```python
from build123d import *

# Parameters (mm, degrees)
SKETCH1_W           = 107.199818646
SKETCH1_H           = 66.816994634
BOSS_EXTRUDE1_DEPTH = 15
SKETCH2_R           = 8.587881919
BOSS_EXTRUDE2_DEPTH = 15
SKETCH3_R           = 13.34182577
BOSS_EXTRUDE3_DEPTH = 80
SKETCH4_R           = 8.5
CUT_EXTRUDE1_DEPTH  = 110
SKETCH5_R           = 10.65
CUT_EXTRUDE2_DEPTH  = 30


with BuildPart() as part:
    # Sketch1 → Boss-Extrude1 (new, symmetric)
    with BuildSketch(Plane.XY):
        Rectangle(SKETCH1_W, SKETCH1_H)
    extrude(amount=BOSS_EXTRUDE1_DEPTH, both=True)

    # Sketch2 → Boss-Extrude2 (add)
    with BuildSketch(Plane(origin=(0, 33.408497317, 0), x_dir=(1, 0, 0), z_dir=(0, 1, 0))):
        with Locations(Location((0, 0, 0), (0, 0, 90))):
            Circle(SKETCH2_R)
    extrude(amount=BOSS_EXTRUDE2_DEPTH)

    # Sketch3 → Boss-Extrude3 (add)
    with BuildSketch(Plane(origin=(0, 48.408497317, 0), x_dir=(1, 0, 0), z_dir=(0, 1, 0))):
        with Locations(Location((0, 0, 0), (0, 0, 270))):
            Circle(SKETCH3_R)
    extrude(amount=BOSS_EXTRUDE3_DEPTH)

    # Sketch4 → Cut-Extrude1 (cut)
    with BuildSketch(Plane.ZY.offset(53.599909323)):
        with Locations((0, -17.285411507)):
            Circle(SKETCH4_R)
    extrude(amount=-CUT_EXTRUDE1_DEPTH, mode=Mode.SUBTRACT)

    # Sketch5 → Cut-Extrude2 (cut)
    with BuildSketch(Plane(origin=(0, 0, -15), x_dir=(-1, 0, 0), z_dir=(0, 0, -1))):
        Circle(SKETCH5_R)
    extrude(amount=-CUT_EXTRUDE2_DEPTH, mode=Mode.SUBTRACT)


solid = part.part
```
Can you work these out from the model? Positions are in its coordinate system, mm. A direction names the side the tool comes from. Give positions to 0.01 mm unless a question says otherwise; leave off trailing zeros. Order: outer loops, then holes, each group sorted by start corner. A loop starts at its lowest first (then second) coordinate and runs counter-clockwise, first axis right, second up. Notation, with made-up numbers: (69.5, -1) - (92.5, -1) arc R30 ccw to (92.5, 38) - close; hole circle Ø9 at (-34.5, -1). An arc over 180 degrees is marked (long way). Use a Markdown table: item, result. Add a question column.
Q1. Please list where these lines run through material, in increasing order: line 1 along Y through (x, z) = (24, 0); line 2 along Y through (x, z) = (30.5, 10); line 3 along X through (y, z) = (2.5, 7.5).
Q2. If we section it at C-C on x = 0: Write out the boundary of the cut face in (y, z), plus the area to 3 significant figures.
Q3. On a 3-axis mill with a long thin cutter (end or side, diameter ignored), from which of +Z, -Z, +X, -X, +Y, -Y can I reach the whole of each face in a straight line? I mean faces 1 (the flat face through (-9, 48.408, 0)), 2 (the cylindrical face through (-5.11, 87.848, 12.324)), 3 (the flat face through (-13, 0, 15)). Say none if no direction works.
Q4. If we mould it in two halves opening along X, with no side actions, what happens to faces 4 (the cylindrical face through (1.39, 10.56, -0.21)), 5 (the cylindrical face through (8.384, 40.803, 1.862)), 6 (the flat face through (-1, 33.408, -10)), 7 (the flat face through (-53.6, 0, 0))? For each: released by +X, released by -X, zero draft, split by the parting line, or undercut.
Q5. If we section it at D-D on y = 35.5: Write out the boundary of the cut face in (x, z).
Q6. I'm going to push flat-ended pins straight in: pin 1 (10 mm diameter, centred on x = 11.5, z = -9, fed in from +Y); pin 2 (10 mm diameter, centred on y = 95, z = 10.5, fed in from +X); pin 3 (5 mm diameter, centred on x = 12, y = 93.5, fed in from -Z). Where does each tip first touch, or does it pass through?
Q7. If we section it at A-A on y = 0: Write out the boundary of the cut face in (x, z).
Q8. If we section it at B-B on z = 2: Write out the boundary of the cut face in (x, y), plus the area to 3 significant figures.
Answers follow:
| question | item | result |
|---|---|---|
| 1 | line 1 | y = -33.41 to -25.79, -8.79 to 33.41 |
| 1 | line 2 | y = -33.41 to 33.41 |
| 1 | line 3 | x = -53.6 to -10.35, 10.35 to 53.6 |
| 2 | outline | (-33.41, -15) - (-10.65, -15) - (-10.65, -5.31) arc R8.5 cw (long way) to (-10.65, 5.31) - (-10.65, 15) - (-33.41, 15) - close; (10.65, -15) - (33.41, -15) - (33.41, -8.59) - (48.41, -8.59) - (48.41, -13.34) - (128.41, -13.34) - (128.41, 13.34) - (48.41, 13.34) - (48.41, 8.59) - (33.41, 8.59) - (33.41, 15) - (10.65, 15) - close |
| 2 | area | 3,540 mm^2 |
| 3 | face 1 | none |
| 3 | face 2 | +Y |
| 3 | face 3 | +Z, +X, -X, +Y, -Y |
| 4 | face 4 | undercut |
| 4 | face 5 | split by the parting line |
| 4 | face 6 | zero draft |
| 4 | face 7 | released by -X |
| 5 | outline | circle Ø17.18 at (0, 0) |
| 6 | pin 1 | stops at y = 128.41 |
| 6 | pin 2 | stops at x = 12.16 |
| 6 | pin 3 | stops at z = -9.37 |
| 7 | outline | (-53.6, -15) - (-10.65, -15) - (-10.65, 15) - (-53.6, 15) - close; (10.65, -15) - (53.6, -15) - (53.6, 15) - (10.65, 15) - close |
| 8 | outline | (-53.6, -33.41) - (53.6, -33.41) - (53.6, -25.55) - (-53.6, -25.55) - close; (-53.6, -9.02) - (-5.66, -9.02) arc R10.65 cw (long way) to (5.66, -9.02) - (53.6, -9.02) - (53.6, 33.41) - (8.35, 33.41) - (8.35, 48.41) - (13.19, 48.41) - (13.19, 128.41) - (-13.19, 128.41) - (-13.19, 48.41) - (-8.35, 48.41) - (-8.35, 33.41) - (-53.6, 33.41) - close |
| 8 | area | 7,410 mm^2 |
